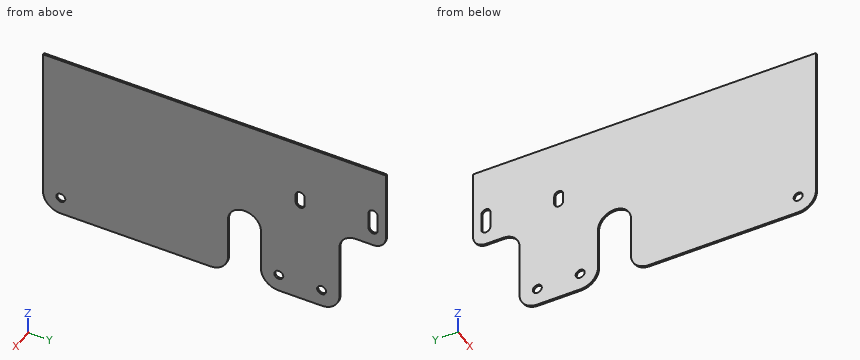
```python
from build123d import *

# Parameters (mm, degrees)
F0_R     = 10.5
F1_DEPTH = 4.5


# Not quite as in the source:
# - a feature names something its author has since deleted; it is built from what else it names


with BuildPart() as f1:
    # F0 (on Right) → F1 (new body)
    with BuildSketch(Plane.YZ):
        with BuildLine():
            Line((-800, -79.2), (-800, -246.5))
            Line((-800, -246.5), (-800, -445))
            ThreePointArc((-800, -445), (-787.8449314192, -474.3449314192), (-758.5, -486.5))
            Line((-758.5, -486.5), (-410, -486.5))
            ThreePointArc((-410, -486.5), (-380.6550685808, -474.3449314192), (-368.5, -445))
            Line((-368.5, -445), (-368.5, -345))
            ThreePointArc((-368.5, -345), (-330, -306.5), (-291.5, -345))
            Line((-291.5, -345), (-291.5, -445))
            ThreePointArc((-291.5, -445), (-279.3449314192, -474.3449314192), (-250, -486.5))
            Line((-250, -486.5), (-150, -486.5))
            ThreePointArc((-150, -486.5), (-120.6550685808, -474.3449314192), (-108.5, -445))
            Line((-108.5, -445), (-108.5, -315))
            ThreePointArc((-108.5, -315), (-97.2236110757, -287.7763889243), (-70, -276.5))
            Line((-70, -276.5), (-30, -276.5))
            ThreePointArc((-30, -276.5), (-8.7867965644, -267.7132034356), (0, -246.5))
            Line((0, -246.5), (0, -79.2))
            Line((0, -79.2), (-800, -79.2))
        make_face()
        with Locations((-758.5, -445)):
            Circle(F0_R, mode=Mode.SUBTRACT)
        with Locations((-250, -445)):
            Circle(F0_R, mode=Mode.SUBTRACT)
        with Locations((-150, -445)):
            Circle(F0_R, mode=Mode.SUBTRACT)
        with BuildLine():
            ThreePointArc((-210.5, -215), (-200, -204.5), (-189.5, -215))
            Line((-189.5, -215), (-189.5, -235))
            ThreePointArc((-189.5, -235), (-200, -245.5), (-210.5, -235))
            Line((-210.5, -235), (-210.5, -215))
        make_face(mode=Mode.SUBTRACT)
        with BuildLine():
            ThreePointArc((-40.5, -195), (-30, -184.5), (-19.5, -195))
            Line((-19.5, -195), (-19.5, -235))
            ThreePointArc((-19.5, -235), (-30, -245.5), (-40.5, -235))
            Line((-40.5, -235), (-40.5, -195))
        make_face(mode=Mode.SUBTRACT)
    extrude(amount=F1_DEPTH)


solid = f1.part
```
Can you work these out from the model? Positions are in its coordinate system, mm. Round coordinates to 2 decimals unless told otherwise and drop trailing zeros. Loops run counter-clockwise (first coordinate to the right, second up) from the corner with the lowest first, then second, coordinate; pieces in that order, holes last. Notation, with made-up numbers: M 55,52 L 72,52 A30 cw 72,77 Z; hole C 69,10 d5. An arc over 180 degrees is marked long. Answer in a Markdown table with one row per item.
1. If we section it at C-C, the plane y = -200: Please give me the cut outline in (x, z), plus the area to 3 significant figures.
Established:
| item | result |
|---|---|
| outline | M 0,-486.5 L 4.5,-486.5 L 4.5,-245.5 L 0,-245.5 Z; M 0,-204.5 L 4.5,-204.5 L 4.5,-79.2 L 0,-79.2 Z |
| area | 1,650 mm² |
2. Please list where these lines run through material, in increasing order: line 1 (Y direction, x = 3.2, z = -344.5); line 2 (Z direction, x = 1.9, y = -150); line 3 (Y direction, x = 3.8, z = -453.5). Write a range as from..to.
Established:
| item | result |
|---|---|
| line 1 | -800..-368.5, -291.5..-108.5 |
| line 2 | -486.5..-455.5, -434.5..-79.2 |
| line 3 | -799.12..-764.66, -752.34..-369.38, -290.62..-256.16, -243.84..-156.16, -143.84..-109.38 |
3. If we section it at A-A, the plane z = -386.5: Please give me the cut outline in (x, y), plus the area to 3 significant figures.
Established:
| item | result |
|---|---|
| outline | M 0,-800 L 4.5,-800 L 4.5,-368.5 L 0,-368.5 Z; M 0,-291.5 L 4.5,-291.5 L 4.5,-108.5 L 0,-108.5 Z |
| area | 2,770 mm² |
4. If we section it at D-D, the plane y = -330: Please give me the cut outline in (x, z), plus the area to 3 significant figures.
Established:
| item | result |
|---|---|
| outline | M 0,-306.5 L 4.5,-306.5 L 4.5,-79.2 L 0,-79.2 Z |
| area | 1,020 mm² |
5. If we section it at B-B, the plane x = 1.9: Please give me the cut outline in (y, z).
Established:
| item | result |
|---|---|
| outline | M -800,-445 A41.5 ccw -758.5,-486.5 L -410,-486.5 A41.5 ccw -368.5,-445 L -368.5,-345 A38.5 cw -291.5,-345 L -291.5,-445 A41.5 ccw -250,-486.5 L -150,-486.5 A41.5 ccw -108.5,-445 L -108.5,-315 A38.5 cw -70,-276.5 L -30,-276.5 A30 ccw 0,-246.5 L 0,-79.2 L -800,-79.2 Z; hole C -758.5,-445 d21; hole C -250,-445 d21; hole M -210.5,-235 A10.5 ccw -189.5,-235 L -189.5,-215 A10.5 ccw -210.5,-215 Z; hole C -150,-445 d21; hole M -40.5,-235 A10.5 ccw -19.5,-235 L -19.5,-195 A10.5 ccw -40.5,-195 Z |
6. I'm going to push a flat-ended pin straight in: pin 1 Ø17 at (y, z) = (-758.5, -445) entering from +X. Where does the tip first touch, or does it pass through?
Established:
| item | result |
|---|---|
| pin 1 | through |
